Could you check a few things on this drawing? It's one solid part, dimensions in mm from its lowest x, y, z. A direction names the side the tool comes from. Give positions to 0.01 mm unless a question says otherwise; leave off trailing zeros. Loops run counter-clockwise (first coordinate to the right, second up) from the corner with the lowest first, then second, coordinate; pieces in that order, holes last.
Q1. I'm going to push flat-ended pins straight in: P1, Ø2.5, axis at x = 6.5, z = 2, coming from the -Y side; P2, Ø1, axis at y = 2.5, z = 9.5, coming from the -X side. Where does each tip first touch, or does it pass through?
Q2. For the marked faces 4, 5 and 6, which set-ups out of +Z, -Z, +X, -X, +Y, -Y let a thin tool reach every point of the face, with its end or its side?
Q3. Suppose I cut it at A-A (y = 15.75). List the corners of the cut face in (x, z) for me, and give its area (3 significant figures).
Q4. Suppose I cut it at C-C (z = 12.25). List the corners of the cut face in (x, y) for me.
Q5. Suppose I cut it at B-B (x = 14.89). List the corners of the cut face in (y, z) for me (1 decimal), and give its area (3 significant figures).
Q6. Thinking about a two-plate mould opening in Z: for the marked faces 1, 2 and 3, which applies, pulls with the +Z half, pulls with the -Z half, needs draft (parallel to the pull), parting line crosses it, or undercut?
Q7. I need wall thicknesses on probe 1 along Z at (x, y) = (8.5, 14.5); probe 2 along X at (y, z) = (19.25, 12.5); probe 3 along Z at (x, y) = (2, 19.25). Which ranges of each line are inside material? Lowest first, please.
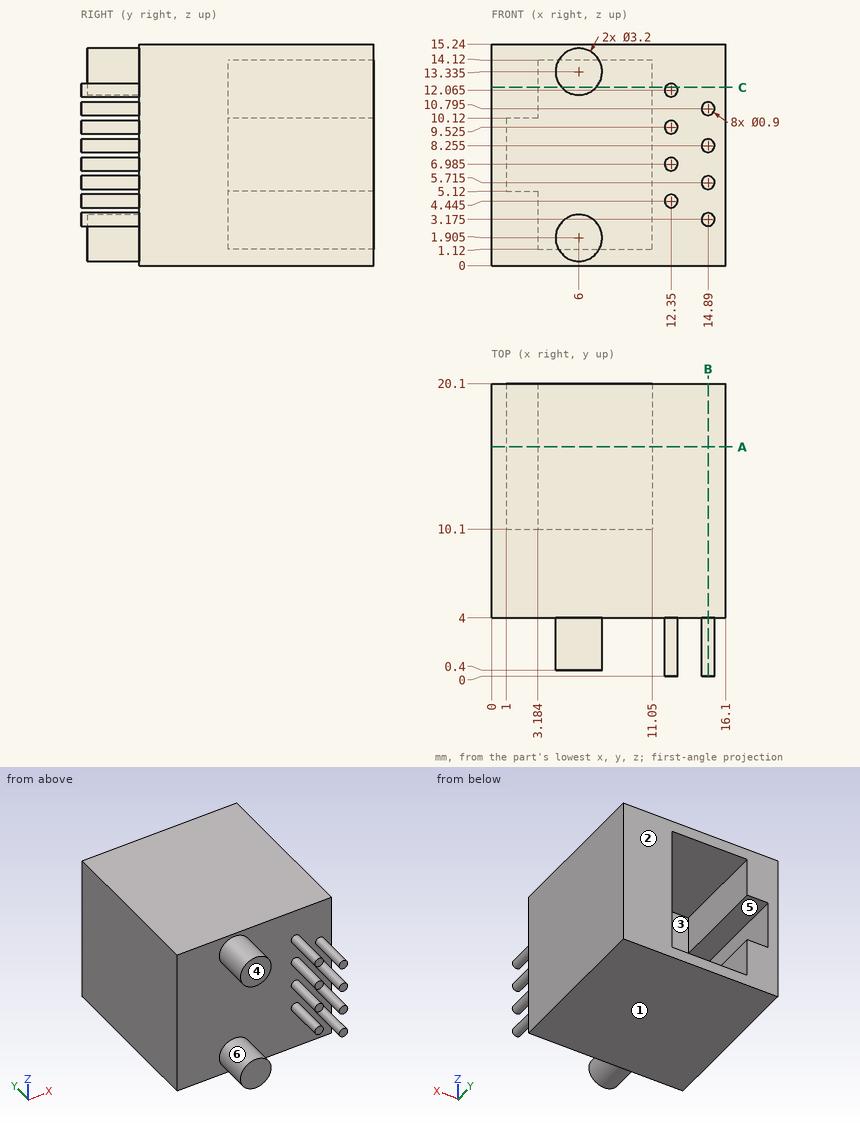
Solutions:
1. P1: stops at y = 0.4
1. P2: stops at x = 11.9
2. face 4: +Z, -Z, -X, -Y
2. face 5: +Y
2. face 6: -Y
3. outline: (0, 0) - (16.1, 0) - (16.1, 15.24) - (0, 15.24) - close; hole (1, 5.12) - (3.18, 5.12) - (3.18, 1.12) - (11.05, 1.12) - (11.05, 14.12) - (3.18, 14.12) - (3.18, 10.12) - (1, 10.12) - close
3. area: 132 mm2
4. outline: (0, 4) - (4.82, 4) - (4.82, 0.4) - (7.18, 0.4) - (7.18, 4) - (11.94, 4) - (11.94, 0) - (12.76, 0) - (12.76, 4) - (16.1, 4) - (16.1, 20.1) - (11.05, 20.1) - (11.05, 10.1) - (3.18, 10.1) - (3.18, 20.1) - (0, 20.1) - close
5. outline: (0, 2.7) - (4, 2.7) - (4, 0) - (20.1, 0) - (20.1, 15.2) - (4, 15.2) - (4, 11.2) - (0, 11.2) - (0, 10.3) - (4, 10.3) - (4, 8.7) - (0, 8.7) - (0, 7.8) - (4, 7.8) - (4, 6.2) - (0, 6.2) - (0, 5.3) - (4, 5.3) - (4, 3.6) - (0, 3.6) - close
5. area: 260 mm2
6. face 1: pulls with the -Z half
6. face 2: needs draft
6. face 3: undercut
7. probe 1: z = 0 to 1.12, 14.12 to 15.24
7. probe 2: x = 0 to 3.18, 11.05 to 16.1
7. probe 3: z = 0 to 5.12, 10.12 to 15.24
